Part model, mm, in its own coordinate system. A direction names the side the tool comes from. Round coordinates to 2 decimals unless told otherwise and drop trailing zeros. Loops run counter-clockwise (first coordinate to the right, second up) from the corner with the lowest first, then second, coordinate; pieces in that order, holes last.
(1) Probe probe 1 along Y at (x, z) = (0.3, -7); probe 2 along X at (y, z) = (5, -22); probe 3 along Z at (x, y) = (0.6, 38). List the from-to ranges inside material, lowest first.
(2) Flat gauge pins, fed straight in: pin 1 (3.5 mm diameter, centred on y = 38, z = -7, fed in from -X); pin 2 (5 mm diameter, centred on y = 29, z = -29.5, fed in from +X); pin 3 (6 mm diameter, centred on x = 11.5, y = 37, fed in from +Z); pin 4 (1 mm diameter, centred on y = 20.5, z = -22, fed in from -X). Where does each tip first touch, or does it go through?
(3) Cut at A-A on z = -7. List the corners of the cut face in (x, y).
(4) Cut at C-C on y = 27. List the corners of the cut face in (x, z).
(5) Cut at B-B on y = 7. List the corners of the cut face in (x, z), then the cut area to 3 significant figures.
(6) Cut at D-D on x = 10.5. List the corners of the cut face in (y, z), then the cut area to 3 significant figures.
(7) Mould opens along Z. For faces 1 (the face through (0.5, 22.2, 0)), 2 (the face through (0.49, 35.77, -6.71)), 3 (the face through (0.3, 0, -22.4)), 4 (the face through (0.6, 22.82, -33.93)) say: +Z half, -Z half, draft (parallel to the pull), parting line (faces both ways), or undercut.
(8) Tool access for faces 5 (the face through (9, 23, -34.5)), 6 (the face through (8, 23, -33.5)): list every direction of +Z, -Z, +X, -X, +Y, -Y with a clear straight run to the whole face (end or side of a thin tool).
Autodesk Inventor part; units mm, degrees
ref_plane "YZ Plane" through (0, 0, 0) normal (1, 0, 0) x (0, 1, 0)
ref_plane "XZ Plane" through (0, 0, 0) normal (0, 1, 0) x (-1, 0, 0)
ref_plane "XY Plane" through (0, 0, 0) normal (0, 0, 1) x (1, 0, 0)
sketch "Sketch1" plane through (0, 0, 0) normal (1, 0, 0) x (0, 1, 0)
  line L0 (0, 0) -> (45, 0)
  line L1 (45, 0) -> (45, -34.5)
  line L2 (45, -34.5) -> (0, -34.5)
  line L3 (0, -34.5) -> (0, 0)
  dimension "d0" = 45
  dimension "d1" = 34.5
extrude "Plate1" add sketch "Sketch1" along normal blind 1
sketch "Sketch2" plane through (0, 45, -33.5) normal (0, 0, -1) x (-1, 0, 0)
  line L0 (0, -45) -> (0, 0)
  line L1 (0, 0) -> (-15, 0)
  line L2 (-15, 0) -> (-15, -45)
  line L3 (-15, -45) -> (0, -45)
edge flange "Flange1" height 15 angle 90 thickness 1 bend radius 1 thickness toward (0, 0, -1) relief tear relief width 1 relief depth 0.5 edges at (1, 22.5, -34.5) wall of the first edge with corners at (0, 0, -33.5) (0, 45, -33.5) (15, 45, -33.5) (15, 0, -33.5)
bend "Bend1"
corner "Corner1"
sketch "Sketch3" plane through (1, 0, 0) normal (1, 0, 0) x (0, 0, -1)
  line L0 (0, 45) -> (32.5, 45)
  line L1 (0, 0) -> (0, 45)
  line L2 (32.5, 0) -> (0, 0)
  point P0 (7, 38)
  point P1 (7, 7)
  dimension "d13" = 7
  dimension "d14" = 7
  dimension "d15" = 7
hole "Hole1" at (1, 38, -7) at (1, 7, -7) direction (-1, 0, 0) diameter 4.5 end through all
equation "\"d21\" = Thickness"
equation "\"d2\" = Thickness"
equation "\"d3\" = BendReliefWidth"
equation "\"d4\" = BendReliefDepth"
equation "\"d5\" = MinimumRemnant"
equation "\"d6\" = TransitionRadius"
equation "\"d9\" = BendRadius"
equation "\"d10\" = CornerReliefSize"
equation "\"d11\" = GapSize"
equation "\"d12\" = JacobiRadiusSize"
equation "\"BendRadius\" = Thickness"
equation "\"BendReliefWidth\" = Thickness"
equation "\"BendReliefDepth\" = 0.5 * Thickness"
equation "\"CornerReliefSize\" = 4 * Thickness"
equation "\"MinimumRemnant\" = 2 * Thickness"
equation "\"TransitionRadius\" = BendRadius"
equation "\"JacobiRadiusSize\" = BendRadius"
equation "\"GapSize\" = Thickness"
properties part number "Plate A connector box-iv stand" material "Steel, Carbon"
Final values:
1. probe 1: y = 0 to 4.75, 9.25 to 35.75, 40.25 to 45
1. probe 2: x = 0 to 1
1. probe 3: z = -33.93 to -9.25, -4.75 to 0
2. pin 1: passes through
2. pin 2: stops at x = 1
2. pin 3: stops at z = -33.5
2. pin 4: stops at x = 0
3. outline: (0, 0) - (1, 0) - (1, 4.75) - (0, 4.75) - close; (0, 9.25) - (1, 9.25) - (1, 35.75) - (0, 35.75) - close; (0, 40.25) - (1, 40.25) - (1, 45) - (0, 45) - close
4. outline: (0, -32.5) arc R2 ccw to (2, -34.5) - (15, -34.5) - (15, -33.5) - (2, -33.5) arc R1 cw to (1, -32.5) - (1, 0) - (0, 0) - close
5. outline: (0, -32.5) arc R2 ccw to (2, -34.5) - (15, -34.5) - (15, -33.5) - (2, -33.5) arc R1 cw to (1, -32.5) - (1, -9.25) - (0, -9.25) - close; (0, -4.75) - (1, -4.75) - (1, 0) - (0, 0) - close
5. area: 43.4 mm2
6. outline: (0, -34.5) - (45, -34.5) - (45, -33.5) - (0, -33.5) - close
6. area: 45.0 mm2
7. face 1: +Z half
7. face 2: undercut
7. face 3: draft
7. face 4: -Z half
8. face 5: -Z, +X, -X, +Y, -Y
8. face 6: +Z, +X, +Y, -Y
